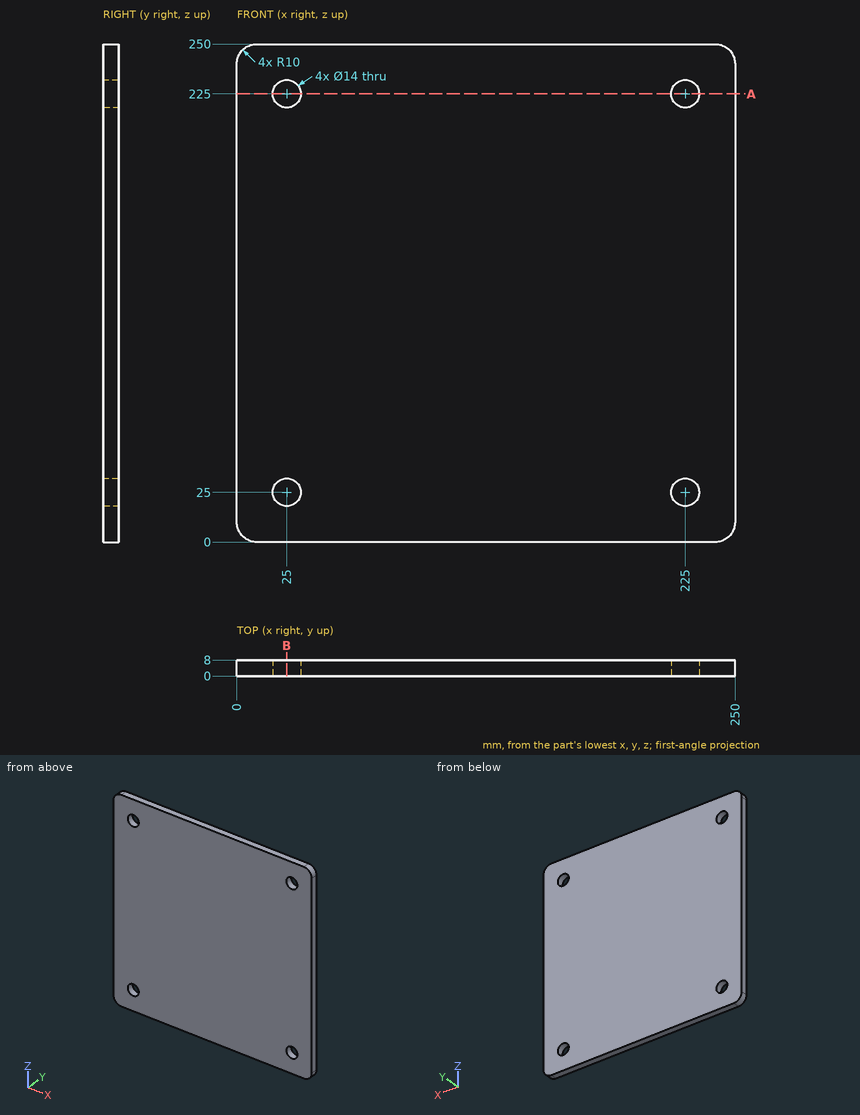
Geometry check sheet. Reference: drawing and pictorial views, mm from the part's lowest x, y, z. Round coordinates to 2 decimals unless told otherwise and drop trailing zeros. Loops run counter-clockwise (first coordinate to the right, second up) from the corner with the lowest first, then second, coordinate; pieces in that order, holes last. Notation, with made-up numbers: (32, 12.5) - (47, 12.5) arc R7 ccw to (47, 18.5) - close; hole circle Ø9 at (53, 56). An arc over 180 degrees is marked (long way). Answer as CSV lines item,"result".
(1) Material ranges on line 1 along X through (y, z) = (3.5, 25); line 2 along X through (y, z) = (7, 23.5); line 3 along Z through (x, y) = (219, 3.25), recorded low to high.
Output values:
line 1,"x = 0 to 18, 32 to 218, 232 to 250"
line 2,"x = 0 to 18.16, 31.84 to 218.16, 231.84 to 250"
line 3,"z = 0 to 21.39, 28.61 to 221.39, 228.61 to 250"
(2) Depth check by flat-ended pin: pin 1 Ø16 at (x, z) = (25, 25) entering from +Y; pin 2 Ø8.5 at (x, z) = (25, 225) entering from +Y. Enter the tip coordinate at first touch or a pass-through.
Output values:
pin 1,"stops at y = 8"
pin 2,"passes through"
(3) Cross-section at B-B, the plane x = 25. Enter the section's corners in (y, z).
Output values:
outline,"(0, 0) - (8, 0) - (8, 18) - (0, 18) - close; (0, 32) - (8, 32) - (8, 218) - (0, 218) - close; (0, 232) - (8, 232) - (8, 250) - (0, 250) - close"
(4) Cross-section at A-A, the plane z = 225. Enter the section's corners in (x, y).
Output values:
outline,"(0, 0) - (18, 0) - (18, 8) - (0, 8) - close; (32, 0) - (218, 0) - (218, 8) - (32, 8) - close; (232, 0) - (250, 0) - (250, 8) - (232, 8) - close"
